```python
from build123d import *

# Parameters (mm, degrees)
PAD_DEPTH    = 4
PAD001_DEPTH = 138
PAD002_DEPTH = 85
POCKET_DEPTH = 10
FILLET_R     = 0.4
FILLET001_R  = 2


with BuildPart() as part:
    # Sketch → Pad (new body)
    with BuildSketch(Plane.XY):
        with BuildLine():
            Line((0, 0), (148, 0))
            Line((148, 0), (148, 113))
            Line((132.604686, 113), (148, 113))
            ThreePointArc((132.604686, 113), (123, 117.5), (113.395314, 113))
            Line((34.604686, 113), (113.395314, 113))
            ThreePointArc((34.604686, 113), (25, 117.5), (15.395314, 113))
            Line((0, 113), (15.395314, 113))
            Line((0, 113), (0, 0))
        make_face()
    extrude(amount=PAD_DEPTH)

    # Sketch001 (on Face3 of Pad) → Pad001 (join)
    with BuildSketch(Plane(origin=(5, 0, 0), x_dir=(0, -1, 0), z_dir=(-1, 0, 0))):
        Polygon((3, 0), (3, -2.5), (-3, -2.5), (-5.5, 0), (0, 0), align=None)
    extrude(amount=-PAD001_DEPTH)

    # Sketch002 (on Face10 of Pad001) → Pad002 (join)
    with BuildSketch(Plane.XZ.offset(-13)):
        with BuildLine():
            Line((143.8, 0), (140.3, 0))
            Line((140.3, 0), (142.3, -6))
            Line((142.3, -6), (143.8, -6))
            ThreePointArc((143.8, -6), (144.65, -5.15), (143.8, -4.3))
            Line((143.8, 0), (143.8, -4.3))
        make_face()
        with BuildLine():
            Line((4.2, 0), (4.2, -4.3))
            ThreePointArc((4.2, -4.3), (3.35, -5.15), (4.2, -6))
            Line((4.2, -6), (5.7, -6))
            Line((5.7, -6), (7.7, 0))
            Line((7.7, 0), (4.2, 0))
        make_face()
    extrude(amount=-PAD002_DEPTH)

    # Sketch003 (on Face4 of Pad002) → Pocket (cut)
    with BuildSketch(Plane(origin=(0, 0, 0), x_dir=(1, 0, 0), z_dir=(0, 0, -1))):
        Polygon((100, 10), (10, 10), (10, -20), (-10, -20), (-10, -43.333333), (10, -43.333333), (10, -66.666667), (-10, -66.666667), (-10, -90), (158, -90), (158, -66.666667), (100, -66.666667), (100, -43.333333), (158, -43.333333), (158, -20), (100, -20), align=None)
    extrude(amount=POCKET_DEPTH, mode=Mode.SUBTRACT)

    # Fillet
    fillet_edges = [part.edges().sort_by_distance(p)[0] for p in [
        (121.5, -3, 0),
        (7.5, -3, 0),
    ]]
    fillet(fillet_edges, radius=FILLET_R)

    # Fillet001
    fillet001_edges = [part.edges().sort_by_distance(p)[0] for p in [
        (0, 56.5, 4),
        (7.697657, 113, 4),
        (25, 117.5, 4),
        (74, 113, 4),
        (148, 56.5, 4),
        (140.302343, 113, 4),
        (123, 117.5, 4),
    ]]
    fillet(fillet001_edges, radius=FILLET001_R)


solid = part.part
```
Work out the finished part from the listing and answer in its coordinate system (mm). A direction names the side the tool comes from. Round coordinates to 2 decimals unless told otherwise and drop trailing zeros. Write each loop counter-clockwise with the first axis right and the second up, starting at its lowest first coordinate (ties: lowest second). Pieces come first, ordered by that corner, then holes.
1) A cutting plane is placed at B-B on x = 54.5. Determine the outline of the cut face in (y, z).
2) Determine the mould class of faces 5 (the face through (141.3, 16.5, -3)), 6 (the face through (73, 60, 0)), 7 (the face through (143.8, 55, -2)), 8 (the face through (73, 59, 4)) for opening direction X: pulls with the +X half, pulls with the -X half, needs draft (parallel to the pull), parting line crosses it, or undercut.
3) Which of the six approach directions +Z, -Z, +X, -X, +Y, -Y give full straight-line access (tool end or side, diameter ignored) to faces 1 (the face through (143.8, 94, -2)), 2 (the face through (141.3, 54.8, -3)), 3 (the face through (142, 90, -3)), 4 (the face through (7, 0, -2.5))?
4) A cutting plane is placed at A-A on y = 40.5. Determine the outline of the cut face in (x, z), and give its area (3 significant figures).
5) Flat-ended cylindrical pins translate along their axes: P1, Ø5, axis at x = 143.5, z = -2.5, coming from the -Y side; P2, Ø6, axis at x = 78, y = 10.5, coming from the -Z side; P3, Ø2, axis at y = 49.5, z = -4.5, coming from the +X side; P4, Ø3.5, axis at x = 142, z = -4, coming from the +Y side. Find the tip coordinate at first contact, or state that the pin passes through.
6) Consider probe 1 along Z at (x, y) = (103, 12); probe 2 along X at (y, z) = (91, -1); probe 3 along Y at (x, z) = (133, -0.5). Determine where each line is inside the solid, lowest interval first.
7) A cutting plane is placed at D-D on y = 54. Determine the outline of the cut face in (x, z).
8) A cutting plane is placed at C-C on x = 110. Determine the outline of the cut face in (y, z), and give its area (3 significant figures).
Entries:
1. outline: (0, 0) - (113, 0) - (113, 2) arc R2 ccw to (111, 4) - (0, 4) - close
2. face 5: undercut
2. face 6: undercut
2. face 7: pulls with the +X half
2. face 8: needs draft
3. face 1: +X, +Y, -Y
3. face 2: -Z, +Y
3. face 3: -Z, +X, -X
3. face 4: -Z, +X, -X, -Y
4. outline: (0, 0) - (148, 0) - (148, 2) arc R2 ccw to (146, 4) - (2, 4) arc R2 ccw to (0, 2) - close
4. area: 590 mm2
5. P1: stops at y = -3
5. P2: stops at z = 0
5. P3: stops at x = 144.65
5. P4: stops at y = 98
6. probe 1: z = 0 to 4
6. probe 2: x = 4.2 to 7.37, 140.63 to 143.8
6. probe 3: y = -3 to 5
7. outline: (0, 0) - (4.2, 0) - (4.2, -4.3) arc R0.85 ccw to (4.2, -6) - (5.7, -6) - (7.7, 0) - (140.3, 0) - (142.3, -6) - (143.8, -6) arc R0.85 ccw to (143.8, -4.3) - (143.8, 0) - (148, 0) - (148, 2) arc R2 ccw to (146, 4) - (2, 4) arc R2 ccw to (0, 2) - close
8. outline: (-3, -2.5) - (3, -2.5) - (5.5, 0) - (113, 0) - (113, 2) arc R2 ccw to (111, 4) - (0, 4) - (0, 0) - (-2.6, 0) arc R0.4 ccw to (-3, -0.4) - close
8. area: 469 mm2
